Build history of the part. All positions in model axes, mm. A direction names the side the tool comes from. Coordinates: 2 decimals unless noted, no trailing zeros. Order: outer loops, then holes, each group sorted by start corner. A loop starts at its lowest first (then second) coordinate and runs counter-clockwise, first axis right, second up. Notation, with made-up numbers: (52, 22) - (65, 22) arc R20 cw to (65, 33) - close; hole circle Ø2 at (2.5, 31). An arc over 180 degrees is marked (long way). One line per item, written item: value.
from build123d import *

# Parameters (mm, degrees)
SKETCH1_R                = 13.2
SKETCH1_R_2              = 10.2
BOSS_EXTRUDE1_DEPTH      = 80
SKETCH2_W                = 3.4
SKETCH2_H                = 3.142664369
CUT_EXTRUDE1_DEPTH       = 10
CIRPATTERN1_COUNT        = 4
MIRROR1_COPY_1_SKETCH_W  = 3.4
MIRROR1_COPY_1_SKETCH_H  = 3.142664369
MIRROR1_COPY_1_DEPTH     = 10
MIRROR1_COPY_2_SKETCH_W  = 3.4
MIRROR1_COPY_2_SKETCH_H  = 3.142664369
MIRROR1_COPY_2_DEPTH     = 10
MIRROR1_COPY_3_SKETCH_W  = 3.4
MIRROR1_COPY_3_SKETCH_H  = 3.142664369
MIRROR1_COPY_3_DEPTH     = 10
BOSS_EXTRUDE3_DEPTH      = 1.5
FILLET1_R                = 6
CIRPATTERN2_COUNT        = 4
FILLET1_OF_CIRPATTERN2_R = 6


with BuildPart() as part:
    # Sketch1 → Boss-Extrude1 (new body)
    with BuildSketch(Plane.XY):
        Circle(SKETCH1_R)
        Circle(SKETCH1_R_2, mode=Mode.SUBTRACT)
    extrude(amount=BOSS_EXTRUDE1_DEPTH)

    # Sketch2 → Cut-Extrude1 (cut)
    with BuildSketch(Plane.XY.offset(80)):
        with Locations((0, 11.628667816)):
            Rectangle(SKETCH2_W, SKETCH2_H)
    cut_extrude1 = extrude(amount=-CUT_EXTRUDE1_DEPTH, mode=Mode.SUBTRACT)

    # CirPattern1: Cut-Extrude1 ×4 about axis
    cirpattern1_axis = Axis((0, 0, 0), (0, 0, 1))
    for i in range(1, CIRPATTERN1_COUNT):
        add(cut_extrude1.rotate(cirpattern1_axis, i * 360 / CIRPATTERN1_COUNT), mode=Mode.SUBTRACT)

    # Mirror1: Cut-Extrude1 across plane
    add(cut_extrude1.mirror(Plane.XY.offset(40)), mode=Mode.SUBTRACT)

    # Mirror1 copy 1 sketch → Mirror1 copy 1 (cut)
    with BuildSketch(Plane.YX):
        with Locations((0, -11.628667816)):
            Rectangle(MIRROR1_COPY_1_SKETCH_W, MIRROR1_COPY_1_SKETCH_H)
    extrude(amount=-MIRROR1_COPY_1_DEPTH, mode=Mode.SUBTRACT)

    # Mirror1 copy 2 sketch → Mirror1 copy 2 (cut)
    with BuildSketch(Plane(origin=(0, 0, 0), x_dir=(-1, 0, 0), z_dir=(0, 0, -1))):
        with Locations((0, -11.628667816)):
            Rectangle(MIRROR1_COPY_2_SKETCH_W, MIRROR1_COPY_2_SKETCH_H)
    extrude(amount=-MIRROR1_COPY_2_DEPTH, mode=Mode.SUBTRACT)

    # Mirror1 copy 3 sketch → Mirror1 copy 3 (cut)
    with BuildSketch(Plane(origin=(0, 0, 0), x_dir=(0, -1, 0), z_dir=(0, 0, -1))):
        with Locations((0, -11.628667816)):
            Rectangle(MIRROR1_COPY_3_SKETCH_W, MIRROR1_COPY_3_SKETCH_H)
    extrude(amount=-MIRROR1_COPY_3_DEPTH, mode=Mode.SUBTRACT)

    # Sketch5 → Boss-Extrude3 (add, symmetric)
    with BuildSketch(Plane(origin=(0, 0, 0), x_dir=(-0.70710678118655, -0.7071067811865451, 0), z_dir=(0.7071067811865451, -0.70710678118655, 0))):
        Polygon((11.2, 0), (13.2, 0), (23.535898385, 0), (27, -6), (27, -74), (23.535898385, -80), (13.2, -80), (11.2, -80), align=None)
    boss_extrude3 = extrude(amount=BOSS_EXTRUDE3_DEPTH, both=True)

    # Fillet1
    fillet1_edges = [part.edges().sort_by_distance(p)[0] for p in [
        (-19.091883092, -19.091883092, 74),
        (-19.091883092, -19.091883092, 6),
    ]]
    fillet(fillet1_edges, radius=FILLET1_R)

    # CirPattern2: Boss-Extrude3 ×4 about axis
    cirpattern2_axis = Axis((0, 0, 0), (0, 0, 1))
    for i in range(1, CIRPATTERN2_COUNT):
        add(boss_extrude3.rotate(cirpattern2_axis, i * 360 / CIRPATTERN2_COUNT))

    # Fillet1 of CirPattern2
    fillet1_of_cirpattern2_edges = [part.edges().sort_by_distance(p)[0] for p in [
        (19.091883092, -19.091883092, 74),
        (19.091883092, -19.091883092, 6),
        (19.091883092, 19.091883092, 74),
        (19.091883092, 19.091883092, 6),
        (-19.091883092, 19.091883092, 74),
        (-19.091883092, 19.091883092, 6),
    ]]
    fillet(fillet1_of_cirpattern2_edges, radius=FILLET1_OF_CIRPATTERN2_R)


solid = part.part
1. Two-plate mould, pull along X, no slides. Class faces 4 (the face through (17.581, 17.611, 77.664)), 5 (the face through (-13.2, 0.1, 39.4)), 6 (the face through (-12, 1.7, 5)), 7 (the face through (-1.7, -12, 75)): pulls with the +X half, pulls with the -X half, needs draft (parallel to the pull), parting line crosses it, or undercut.
Values found:
face 4: pulls with the +X half
face 5: pulls with the -X half
face 6: needs draft
face 7: undercut
2. Band-saw the part on C-C, the plane z = 6. Count the separate pieces of the cut face and the enclosed holes in it, and give its area (3 significant figures).
Values found:
separate pieces: 4
enclosed holes: 0
area: 343 mm2
3. Band-saw the part on A-A, the plane x = 0. Give the cut face in (y, z).
Values found:
outline: (-13.2, 10) - (-10.2, 10) - (-10.2, 70) - (-13.2, 70) - close; (10.2, 10) - (13.2, 10) - (13.2, 70) - (10.2, 70) - close
4. Flat gauge pins, fed straight in: P1, Ø1.5, axis at x = -12, z = 77, coming from the +Y side; P2, Ø2, axis at y = -11, z = 32.5, coming from the -X side; P3, Ø1.6, axis at x = 0, y = -11, coming from the +Z side; P4, Ø18.5, axis at x = 0, y = 0, coming from the +Z side. Where does each tip first touch, or does it go through?
Values found:
P1: stops at y = 14.87
P2: stops at x = -14.12
P3: stops at z = 70
P4: passes through
5. Probe line 1 along X through (y, z) = (0, 50); line 2 along X through (y, z) = (-12, 31.5). List the from-to ranges inside material, lowest first.
Values found:
line 1: x = -13.2 to -10.2, 10.2 to 13.2
line 2: x = -14.12 to -9.88, -5.5 to 5.5, 9.88 to 14.12
6. 3-axis set-ups, long thin cutter, end or side, ignore diameter. For faces 1 (the face through (13.19, 15.31, 39.44)), 2 (the face through (15.31, -13.19, 39.44)), 3 (the face through (-12, -1.7, 5)): which of +Z, -Z, +X, -X, +Y, -Y reach the whole face in a straight line?
Values found:
face 1: +Z, -Z, +Y
face 2: +Z, -Z, +X
face 3: -Z, +X, -X
7. Band-saw the part on D-D, the plane z = 63.5. Give the cut face in (x, y), and give its area (3 significant figures).
Values found:
outline: (-20.15, -18.03) - (-18.03, -20.15) - (-8.21, -10.33) arc R13.2 ccw to (8.21, -10.33) - (18.03, -20.15) - (20.15, -18.03) - (10.33, -8.21) arc R13.2 ccw to (10.33, 8.21) - (20.15, 18.03) - (18.03, 20.15) - (8.21, 10.33) arc R13.2 ccw to (-8.21, 10.33) - (-18.03, 20.15) - (-20.15, 18.03) - (-10.33, 8.21) arc R13.2 ccw to (-10.33, -8.21) - close; hole circle Ø20.4 at (0, 0)
area: 386 mm2
